from build123d import *

# Parameters (mm, degrees)
F1_DEPTH = 22.5
F2_R     = 2.5
F3_DEPTH = 5.001
F4_R     = 2.5
F5_DEPTH = 5.807106


with BuildPart() as f1:
    # F0 (on Front) → F1 (new body)
    with BuildSketch(Plane.XZ):
        with BuildLine():
            Line((-27.208689, 5.806106), (-27.048263, 0))
            Line((-27.048263, 0), (32.951737, 0))
            Line((32.951737, 0), (32.951737, 5))
            Line((32.951737, 5), (20.451737, 5))
            Line((20.451737, 5), (20.451737, 17.5))
            Line((20.451737, 17.5), (15.451737, 17.5))
            ThreePointArc((15.451737, 17.5), (2.955538, 5.308247), (-9.540661, 17.5))
            Line((-9.540661, 17.5), (-14.540661, 17.5))
            Line((-14.540661, 17.5), (-14.540661, 5.806106))
            Line((-14.540661, 5.806106), (-14.708689, 5.806106))
            Line((-14.708689, 5.806106), (-27.208689, 5.806106))
        make_face()
    extrude(amount=F1_DEPTH)

    # F2 (on face) → F3 (cut, through all)
    with BuildSketch(Plane.XY.offset(5)):
        with Locations((26.701737, -11.25)):
            Circle(F2_R)
    extrude(amount=-F3_DEPTH, mode=Mode.SUBTRACT)

    # F4 (on face) → F5 (cut, through all)
    with BuildSketch(Plane.XY.offset(5.806106)):
        with Locations((-20.874675, -11.25)):
            Circle(F4_R)
    extrude(amount=-F5_DEPTH, mode=Mode.SUBTRACT)


solid = f1.part
Design review of the part built by this model. Coordinates are the model's own, in mm. A direction names the side the tool comes from. Give positions to 0.01 mm unless a question says otherwise; leave off trailing zeros. Loops run counter-clockwise (first coordinate to the right, second up) from the corner with the lowest first, then second, coordinate; pieces in that order, holes last. Notation, with made-up numbers: M 54,-7 L 61,-7 A31 ccw 61,26 Z; hole C 41,28 d7. An arc over 180 degrees is marked long. One line per question, with ' | ' between items. Start each with the question number.
1. Add section B-B (z = 9.5). Write out the cut boundary in (x, y), plus the area to 3 significant figures.
2. Add section C-C (y = -15.75). Write out the cut boundary in (x, z).
3. Insertion check: P1, Ø6.5, axis at x = -20.87, y = -11.25, coming from the +Z side; P2, Ø6, axis at x = 26, y = -9, coming from the +Z side; P3, Ø2, axis at x = 9.5, y = -15.5, coming from the +Z side. Each pin has a flat end and moves straight along its axis. Give the tip position at first contact, or say it passes through.
4. Add section A-A (y = -11.25). Write out the cut boundary in (x, z), plus the area to 3 significant figures.
5. Add section D-D (z = 2.25). Write out the cut boundary in (x, y), plus the area to 3 significant figures.
6. The part is to be moulded in two halves that separate along X. For faces 4 (the face through (3.23, -11.09, 5.31)), 5 (the face through (3, -11, 0)), 6 (the face through (32.952, -11, 2)), 7 (the face through (-14.541, -11, 12)), say which applies: released by +X, released by -X, zero draft, split by the parting line, or undercut.
7. For faces 1 (the face through (-20.8, -8.6, 5.806)), 2 (the face through (26.2, -13.7, 2.5)), 3 (the face through (20.452, -11, 11)), list the 3-axis set-ups (+Z, -Z, +X, -X, +Y, -Y) from which the entire face can be reached by the end or side of a thin tool; tool diameter is ignored.
8. To check wall thickness, follow L1, parallel to X at y = -13.5, z = 4.5; L2, parallel to Y at x = -20.5, z = 2.5; L3, parallel to Z at x = -19, y = -20.75. State the ranges of each line that lie inside material, in increasing order.
Worked out:
1) outline: M -14.54,-22.5 L -6.38,-22.5 L -6.38,0 L -14.54,0 Z; M 12.29,-22.5 L 20.45,-22.5 L 20.45,0 L 12.29,0 Z | area: 367 mm²
2) outline: M -27.21,5.81 L -27.05,0 L 32.95,0 L 32.95,5 L 20.45,5 L 20.45,17.5 L 15.45,17.5 A12.5 cw -9.54,17.5 L -14.54,17.5 L -14.54,5.81 Z
3) P1: stops at z = 5.81 | P2: stops at z = 5 | P3: stops at z = 7.84
4) outline: M -27.21,5.81 L -27.05,0 L -23.37,0 L -23.37,5.81 Z; M -18.37,0 L 24.2,0 L 24.2,5 L 20.45,5 L 20.45,17.5 L 15.45,17.5 A12.5 cw -9.54,17.5 L -14.54,17.5 L -14.54,5.81 L -18.37,5.81 Z; M 29.2,0 L 32.95,0 L 32.95,5 L 29.2,5 Z | area: 456 mm²
5) outline: M -27.11,-22.5 L 32.95,-22.5 L 32.95,0 L -27.11,0 Z; hole C -20.87,-11.25 d5; hole C 26.7,-11.25 d5 | area: 1,310 mm²
6) face 4: undercut | face 5: zero draft | face 6: released by +X | face 7: released by -X
7) face 1: +Z, -X, +Y, -Y | face 2: +Z, -Z | face 3: +Z, +X, +Y, -Y
8) L1: x = -27.17 to -21.96, -19.78 to 25.61, 27.79 to 32.95 | L2: y = -22.5 to -13.72, -8.78 to 0 | L3: z = 0 to 5.81
